The model under review builds one solid part; all positions refer to its coordinate system, in mm. Round coordinates to 2 decimals unless told otherwise and drop trailing zeros. Order: outer loops, then holes, each group sorted by start corner. A loop starts at its lowest first (then second) coordinate and runs counter-clockwise, first axis right, second up.
1) Consider section A-A (z = 0). Give the boundary of the cut face in (x, y).
2) To check wall thickness, follow L1, parallel to Z at x = 300, y = 4.25; L2, parallel to X at y = 5.25, z = -16. State the ranges of each line that lie inside material, in increasing order.
3) Clearance check with flat-ended pins moving along their axes: P1, Ø3, axis at y = 2, z = -7.5, coming from the -X side; P2, Ø1.5, axis at y = 1, z = 20.5, coming from the -X side. State where each tip first meets the part, or that it passes through.
4) Consider section B-B (x = 390). Give the boundary of the cut face in (y, z).
from build123d import *

# Parameters (mm, degrees)
BOSS_EXTRUDE1_DEPTH = 9


with BuildPart() as part:
    # Sketch1 → Boss-Extrude1 (new body)
    # profile 1 of 2: a face of its own
    with BuildSketch(Plane(origin=(0, 0, 0), x_dir=(1, 0, 0), z_dir=(0, 1, 0))):
        with BuildLine():
            Line((0, 30.65), (450, 30.65))
            ThreePointArc((450, 30.65), (480.65, 0), (450, -30.65))
            Line((450, -30.65), (0, -30.65))
            ThreePointArc((0, -30.65), (-30.65, 0), (0, 30.65))
        make_face()
        with BuildLine():
            ThreePointArc((450, -28.65), (478.65, 0), (450, 28.65))
            Line((450, 28.65), (0, 28.65))
            ThreePointArc((0, 28.65), (-28.65, 0), (0, -28.65))
            Line((0, -28.65), (450, -28.65))
        make_face(mode=Mode.SUBTRACT)
    # profile 2 of 2: a face of its own
    with BuildSketch(Plane(origin=(0, 0, 0), x_dir=(1, 0, 0), z_dir=(0, 1, 0))):
        with BuildLine():
            Line((0, -28.65), (450, -28.65))
            ThreePointArc((450, -28.65), (478.65, 0), (450, 28.65))
            Line((450, 28.65), (0, 28.65))
            ThreePointArc((0, 28.65), (-28.65, 0), (0, -28.65))
        make_face()
        with BuildLine():
            ThreePointArc((0, 27.15), (-27.15, 0), (0, -27.15))
            Line((0, -27.15), (450, -27.15))
            ThreePointArc((450, -27.15), (477.15, 0), (450, 27.15))
            Line((450, 27.15), (0, 27.15))
        make_face(mode=Mode.SUBTRACT)
    extrude(amount=BOSS_EXTRUDE1_DEPTH)


solid = part.part
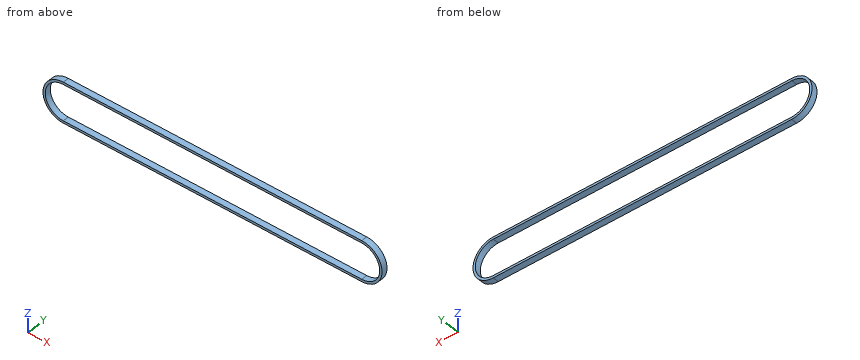
Answer below:
1. outline: (-30.65, 0) - (-27.15, 0) - (-27.15, 9) - (-30.65, 9) - close; (477.15, 0) - (480.65, 0) - (480.65, 9) - (477.15, 9) - close
2. L1: z = -30.65 to -27.15, 27.15 to 30.65
2. L2: x = -26.14 to -21.93, 471.93 to 476.14
3. P1: stops at x = -30.06
3. P2: stops at x = -23.44
4. outline: (0, -30.65) - (9, -30.65) - (9, -27.15) - (0, -27.15) - close; (0, 27.15) - (9, 27.15) - (9, 30.65) - (0, 30.65) - close
